Input: part model. Units: mm. Frame: model coordinates. Face numbers are marked on the shaded views. A direction names the side the tool comes from. Give positions to 0.01 mm unless a question says otherwise; leave off trailing zeros. Order: outer loops, then holes, each group sorted by start corner. A loop starts at its lowest first (then second) coordinate and runs counter-clockwise, first axis right, second up. Notation, with made-up numbers: (-26, 17) - (33, 17) arc R19 ccw to (33, 30) - close; hole circle Ø6 at (-5, -17). An arc over 180 degrees is marked (long way). Answer in a Markdown table with one row per item. Add a question column.
from build123d import *

# Parameters (mm, degrees)
SKETCH1_W           = 282.5
SKETCH1_H           = 105
BOSS_EXTRUDE1_DEPTH = 150.5
SKETCH2_W           = 155
SKETCH2_H           = 105
CUT_EXTRUDE1_DEPTH  = 45.5
SKETCH3_W           = 50
SKETCH3_H           = 50
CUT_EXTRUDE2_DEPTH  = 85
SKETCH4_R           = 5
CUT_EXTRUDE3_DEPTH  = 50
SKETCH5_R           = 5
CUT_EXTRUDE4_DEPTH  = 50
CUT_EXTRUDE5_DEPTH  = 106
CUT_EXTRUDE6_DEPTH  = 106
SKETCH8_R           = 5
CUT_EXTRUDE7_DEPTH  = 50
CUT_EXTRUDE8_DEPTH  = 50
SKETCH10_R          = 5
CUT_EXTRUDE9_DEPTH  = 106
SKETCH11_R          = 5
CUT_EXTRUDE10_DEPTH = 106
SKETCH12_W          = 85
SKETCH12_H          = 85
CUT_EXTRUDE11_DEPTH = 106
SKETCH13_W          = 40
SKETCH13_H          = 32.5
CUT_EXTRUDE12_DEPTH = 151.5
SKETCH14_W          = 20
SKETCH14_H          = 20
CUT_EXTRUDE13_DEPTH = 151.5
CUT_EXTRUDE14_DEPTH = 106
FILLET1_R           = 10
FILLET2_R           = 10
FILLET3_R           = 10


with BuildPart() as part:
    # Sketch1 → Boss-Extrude1 (new body)
    with BuildSketch(Plane(origin=(0, 0, 0), x_dir=(1, 0, 0), z_dir=(0, 1, 0))):
        with Locations((-141.25, -52.5)):
            Rectangle(SKETCH1_W, SKETCH1_H)
    extrude(amount=BOSS_EXTRUDE1_DEPTH)

    # Sketch2 → Cut-Extrude1 (cut)
    with BuildSketch(Plane(origin=(0, 150.5, 0), x_dir=(1, 0, 0), z_dir=(0, 1, 0))):
        with Locations((-205, -52.5)):
            Rectangle(SKETCH2_W, SKETCH2_H)
    extrude(amount=-CUT_EXTRUDE1_DEPTH, mode=Mode.SUBTRACT)

    # Sketch3 → Cut-Extrude2 (cut)
    with BuildSketch(Plane(origin=(0, 105, 0), x_dir=(1, 0, 0), z_dir=(0, 1, 0))):
        with Locations((-152.5, -80)):
            Rectangle(SKETCH3_W, SKETCH3_H)
        with Locations((-152.5, -25)):
            Rectangle(SKETCH3_W, SKETCH3_H)
    extrude(amount=-CUT_EXTRUDE2_DEPTH, mode=Mode.SUBTRACT)

    # Sketch4 → Cut-Extrude3 (cut)
    with BuildSketch(Plane.XY.offset(105)):
        with Locations((-162.5, 10)):
            Circle(SKETCH4_R)
        with BuildLine():
            Line((-152.5, 6), (-127.5, 6))
            Line((-127.5, 6), (-127.5, 105))
            Line((-127.5, 105), (-177.5, 105))
            Line((-177.5, 105), (-177.5, 20))
            Line((-177.5, 20), (-162.5, 20))
            ThreePointArc((-162.5, 20), (-155.428932188, 17.071067812), (-152.5, 10))
            Line((-152.5, 10), (-152.5, 6))
        make_face()
    extrude(amount=-CUT_EXTRUDE3_DEPTH, mode=Mode.SUBTRACT)

    # Sketch5 → Cut-Extrude4 (cut)
    with BuildSketch(Plane(origin=(0, 0, 0), x_dir=(-1, 0, 0), z_dir=(0, 0, -1))):
        with Locations((162.5, 10)):
            Circle(SKETCH5_R)
        with BuildLine():
            Line((127.5, 105), (177.5, 105))
            Line((177.5, 105), (177.5, 20))
            Line((177.5, 20), (162.5, 20))
            ThreePointArc((162.5, 20), (155.428932188, 17.071067812), (152.5, 10))
            Line((152.5, 10), (152.5, 6))
            Line((152.5, 6), (127.5, 6))
            Line((127.5, 6), (127.5, 105))
        make_face()
    extrude(amount=-CUT_EXTRUDE4_DEPTH, mode=Mode.SUBTRACT)

    # Sketch6 → Cut-Extrude5 (cut, through all)
    with BuildSketch(Plane.XY.offset(105)):
        Polygon((0, 40), (-91.138168804, 40), (-124.702154051, 0), (0, 0), align=None)
    extrude(amount=-CUT_EXTRUDE5_DEPTH, mode=Mode.SUBTRACT)

    # Sketch7 → Cut-Extrude6 (cut, through all)
    with BuildSketch(Plane.XY.offset(105)):
        Polygon((-127.5, 105), (-105.130575467, 105), (-66.951542249, 150.5), (-127.5, 150.5), align=None)
    extrude(amount=-CUT_EXTRUDE6_DEPTH, mode=Mode.SUBTRACT)

    # Sketch8 → Cut-Extrude7 (cut)
    with BuildSketch(Plane.XY.offset(105)):
        with Locations((-50, 50)):
            Circle(SKETCH8_R)
        with BuildLine():
            Line((-40, 150.5), (-66.951542249, 150.5))
            Line((-66.951542249, 150.5), (-105.130575467, 105))
            Line((-105.130575467, 105), (-127.5, 105))
            Line((-127.5, 105), (-127.5, 6))
            Line((-127.5, 6), (-93.936014753, 46))
            Line((-93.936014753, 46), (-60, 46))
            Line((-60, 46), (-60, 50))
            ThreePointArc((-60, 50), (-57.071067812, 57.071067812), (-50, 60))
            Line((-50, 60), (-40, 60))
            Line((-40, 60), (-40, 150.5))
        make_face()
    extrude(amount=-CUT_EXTRUDE7_DEPTH, mode=Mode.SUBTRACT)

    # Sketch9 → Cut-Extrude8 (cut)
    with BuildSketch(Plane(origin=(0, 0, 0), x_dir=(-1, 0, 0), z_dir=(0, 0, -1))):
        with BuildLine():
            Line((66.951542249, 150.5), (40, 150.5))
            Line((40, 150.5), (40, 60))
            Line((40, 60), (50, 60))
            ThreePointArc((50, 60), (57.071067812, 57.071067812), (60, 50))
            Line((60, 50), (60, 46))
            Line((60, 46), (93.936014753, 46))
            Line((93.936014753, 46), (127.5, 6))
            Line((127.5, 6), (127.5, 105))
            Line((127.5, 105), (105.130575467, 105))
            Line((105.130575467, 105), (66.951542249, 150.5))
        make_face()
    extrude(amount=-CUT_EXTRUDE8_DEPTH, mode=Mode.SUBTRACT)

    # Sketch10 → Cut-Extrude9 (cut, through all)
    with BuildSketch(Plane(origin=(0, 0, 0), x_dir=(-1, 0, 0), z_dir=(0, 0, -1))):
        with Locations((50, 50)):
            Circle(SKETCH10_R)
    extrude(amount=-CUT_EXTRUDE9_DEPTH, mode=Mode.SUBTRACT)

    # Sketch11 → Cut-Extrude10 (cut, through all)
    with BuildSketch(Plane(origin=(0, 0, 0), x_dir=(-1, 0, 0), z_dir=(0, 0, -1))):
        with Locations((162.5, 10)):
            Circle(SKETCH11_R)
    extrude(amount=-CUT_EXTRUDE10_DEPTH, mode=Mode.SUBTRACT)

    # Sketch12 → Cut-Extrude11 (cut, through all)
    with BuildSketch(Plane(origin=(0, 105, 0), x_dir=(1, 0, 0), z_dir=(0, 1, 0))):
        with Locations((-230, -52.5)):
            Rectangle(SKETCH12_W, SKETCH12_H)
    extrude(amount=-CUT_EXTRUDE11_DEPTH, mode=Mode.SUBTRACT)

    # Sketch13 → Cut-Extrude12 (cut, through all)
    with BuildSketch(Plane(origin=(0, 150.5, 0), x_dir=(1, 0, 0), z_dir=(0, 1, 0))):
        with Locations((-20, -88.75)):
            Rectangle(SKETCH13_W, SKETCH13_H)
        with Locations((-20, -16.25)):
            Rectangle(SKETCH13_W, SKETCH13_H)
    extrude(amount=-CUT_EXTRUDE12_DEPTH, mode=Mode.SUBTRACT)

    # Sketch14 → Cut-Extrude13 (cut, through all)
    with BuildSketch(Plane(origin=(0, 150.5, 0), x_dir=(1, 0, 0), z_dir=(0, 1, 0))):
        with Locations((-20, -52.5)):
            Rectangle(SKETCH14_W, SKETCH14_H)
    extrude(amount=-CUT_EXTRUDE13_DEPTH, mode=Mode.SUBTRACT)

    # Sketch15 → Cut-Extrude14 (cut, through all)
    with BuildSketch(Plane(origin=(0, 105, 0), x_dir=(1, 0, 0), z_dir=(0, 1, 0))):
        Polygon((-224, 0), (-20, -32.5), (-20, 0), align=None)
        Polygon((-224, -105), (-20, -72.5), (-20, -105), align=None)
    extrude(amount=-CUT_EXTRUDE14_DEPTH, mode=Mode.SUBTRACT)

    # Fillet1
    fillet1_edges = [part.edges().sort_by_distance(p)[0] for p in [
        (-93.936014753, 46, 69.639510979),
        (-93.936014753, 46, 35.360489021),
        (-127.5, 6, 72.313112745),
        (-127.5, 6, 32.686887255),
    ]]
    fillet(fillet1_edges, radius=FILLET1_R)

    # Fillet2
    fillet2_edges = [part.edges().sort_by_distance(p)[0] for p in [
        (-124.702154051, 0, 52.5),
        (-91.138168804, 40, 52.5),
    ]]
    fillet(fillet2_edges, radius=FILLET2_R)

    # Fillet3
    fillet3_edges = [part.edges().sort_by_distance(p)[0] for p in [
        (-105.130575467, 105, 52.5),
        (-66.951542249, 150.5, 52.5),
    ]]
    fillet(fillet3_edges, radius=FILLET3_R)


solid = part.part
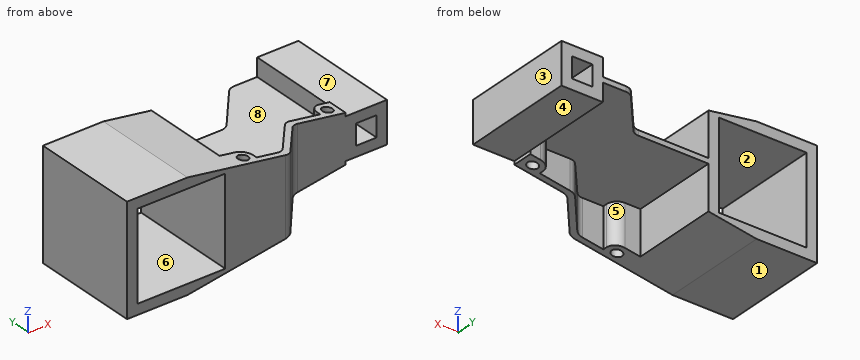
Q1. Access query for the marked faces 4, 5, 6, 7 and 8. Directions: +Z, -Z, +X, -X, +Y, -Y. A direction counts if a zero-diameter tool reaches every point of the face in a straight line with its end or side. Return the directions, or none.
Q2. Pull-direction query (Z, two-part tool) for the marked faces 1, 2 and 3; classes: +Z half, -Z half, draft (parallel to the pull), parting line (faces both ways), or undercut.
Q3. Line query: probe 1 along X at (y, z) = (50, 46); probe 2 along X at (y, z) = (89, 44.5); probe 3 along X at (y, z) = (50, 37.5). Output: solid intervals per line, ascending.
Q4. Section D-D, the plane y = 131. Return loops of the section in (x, z), then the cut area to 3 significant figures.
Q5. Section A-A, the plane y = 86. Return loops of the section in (x, z).
Q6. Section C-C, the plane x = -113. Return loops of the section in (y, z), then the cut area to 3 significant figures.
Q7. Contact query for flat-ended pins moving along their axis: P1, Ø12, axis at x = -171, z = 31, coming from the +Y side; P2, Ø2, axis at x = -123, y = 26.5, coming from the +Z side; P3, Ø12, axis at x = -110, z = 88, coming from the +Y side. Output: stop coordinate, or through.
Q8. Section B-B, the plane y = 24. Return loops of the section in (x, z).
Computed:
| question | item | result |
|---|---|---|
| 1 | face 4 | -Z, +X, +Y, -Y |
| 1 | face 5 | -Z, +Y |
| 1 | face 6 | +Y, -Y |
| 1 | face 7 | +Z, +X, +Y, -Y |
| 1 | face 8 | +Z, +Y |
| 2 | face 1 | -Z half |
| 2 | face 2 | undercut |
| 2 | face 3 | draft |
| 3 | probe 1 | x = -282.5 to -272.5, -187.5 to -177.5, -60 to -55, -45 to -30, -10 to 0 |
| 3 | probe 2 | x = -282.5 to -272.5, -187.5 to -177.5, -40 to -30, -10 to 0 |
| 3 | probe 3 | x = -282.5 to -272.5, -187.5 to -177.5, -60 to -55, -45 to 0 |
| 4 | outline | (-83.31, 50) - (-40, 50) - (-40, 32.5) - (0, 32.5) - (0, 72.5) - (-40, 72.5) - (-40, 55) - (-83.31, 55) - close; hole (-30, 42.5) - (-10, 42.5) - (-10, 62.5) - (-30, 62.5) - close |
| 4 | area | 1,420 mm^2 |
| 5 | outline | (-282.5, 0) - (-224, 0) - (-177.5, 7.41) - (-177.5, 50) - (-40, 50) - (-40, 32.5) - (0, 32.5) - (0, 72.5) - (-40, 72.5) - (-40, 55) - (-177.5, 55) - (-177.5, 97.59) - (-224, 105) - (-282.5, 105) - close; hole (-272.5, 10) - (-187.5, 10) - (-187.5, 95) - (-272.5, 95) - close; hole (-30, 42.5) - (-10, 42.5) - (-10, 62.5) - (-30, 62.5) - close |
| 6 | outline | (13.95, 17.68) - (23.28, 17.68) - (23.28, 50) - (105, 50) - (105, 55) - (23.28, 55) - (23.28, 87.32) - (13.95, 87.32) - close |
| 6 | area | 1,060 mm^2 |
| 7 | P1 | stops at y = 20 |
| 7 | P2 | stops at z = 55 |
| 7 | P3 | stops at y = 33.57 |
| 8 | outline | (-282.5, 0) - (-224, 0) - (-177.5, 7.41) - (-177.5, 50) - (-112.4, 50) - (-112.4, 17.78) - (-104.56, 19.03) - (-104.56, 85.97) - (-112.4, 87.22) - (-112.4, 55) - (-177.5, 55) - (-177.5, 97.59) - (-224, 105) - (-282.5, 105) - close; hole (-272.5, 10) - (-187.5, 10) - (-187.5, 95) - (-272.5, 95) - close |
